The listing builds one solid part. Answer for the finished solid, in the listing's coordinates (mm). A direction names the side the tool comes from. Coordinates: 2 decimals unless noted, no trailing zeros. Write each loop counter-clockwise with the first axis right and the second up, starting at its lowest first coordinate (ties: lowest second). Pieces come first, ordered by that corner, then holes.
(1) Given P1, Ø2, axis at x = -7, y = 7.5, coming from the -Z side; P2, Ø1, axis at x = -7, z = 24, coming from the +Y side; P3, Ø1.3, axis at y = -4, z = 24, coming from the +X side; P4, Ø7, axis at x = -25, z = -3, coming from the -Y side, each flat-ended and moving along its own axis, determine where each tip first touches the part or whether it passes through.
(2) Which of the six approach directions +Z, -Z, +X, -X, +Y, -Y give full straight-line access (tool end or side, diameter ignored) to faces 1 (the flat face through (25, 0, 0)), 2 (the flat face through (0, 10.16, -19)), 3 (the cylindrical face through (0.827, 1.216, -24.148)), 4 (the flat face through (-7, 2.54, 24)), 5 (the flat face through (0, 10.16, 19))?
(3) Straight lines are drawn through the part: line 1 (Y direction, x = 0, z = 23.9); line 2 (X direction, y = 6.25, z = -5) (3 decimals); line 3 (Z direction, x = 6.5, y = -2). For each, find the intervals that lie inside material, in ascending order.
(4) The part is cut by section A-A on y = 5.5. Determine the outline of the cut face in (x, z) (3 decimals).
(5) For a pull along X with two mould halves and no side action, classify faces 6 (the flat face through (6.35, 6, 0)), 7 (the flat face through (-28, 2.54, 0)), 8 (the flat face through (-27.305, 8, 0)) as +X half, -X half, draft (parallel to the pull), parting line (faces both ways), or undercut.
(6) The part is cut by section C-C on z = 11.5. Determine the outline of the cut face in (x, y) (3 decimals).
(7) The part is cut by section D-D on y = -5.08. Determine the outline of the cut face in (x, z).
(8) The part is cut by section B-B on x = 0. Determine the outline of the cut face in (y, z), plus the area to 3 significant figures.
from build123d import *

# Parameters (mm, degrees)
SKETCH1_W           = 57.15
SKETCH1_H           = 25.4
BOSS_EXTRUDE1_DEPTH = 15.24
SKETCH2_W           = 44.45
SKETCH2_H           = 25.4
CUT_EXTRUDE1_DEPTH  = 10.16
SKETCH3_W           = 1.27
SKETCH3_H           = 10.16
CUT_EXTRUDE2_DEPTH  = 42.157602275
BOSS_EXTRUDE2_START = -10.16
SKETCH4_W           = 12.7
SKETCH4_H           = 50.8
BOSS_EXTRUDE2_DEPTH = 7.62
SKETCH6_W           = 15.24
SKETCH6_H           = 15.24
SKETCH6_R           = 6.35
BOSS_EXTRUDE3_DEPTH = 2.54


with BuildPart() as part:
    # Sketch1 → Boss-Extrude1 (new body)
    with BuildSketch(Plane(origin=(0, 0, 0), x_dir=(1, 0, 0), z_dir=(0, 1, 0))):
        Rectangle(SKETCH1_W, SKETCH1_H)
    extrude(amount=BOSS_EXTRUDE1_DEPTH)

    # Sketch2 → Cut-Extrude1 (cut)
    with BuildSketch(Plane.XZ):
        Rectangle(SKETCH2_W, SKETCH2_H)
    extrude(amount=-CUT_EXTRUDE1_DEPTH, mode=Mode.SUBTRACT)

    # Sketch3 → Cut-Extrude2 (cut, through all)
    with BuildSketch(Plane.XY.offset(12.7)):
        with Locations((-27.94, 7.62)):
            Rectangle(SKETCH3_W, SKETCH3_H)
        with Locations((27.94, 7.62)):
            Rectangle(SKETCH3_W, SKETCH3_H)
    extrude(amount=-CUT_EXTRUDE2_DEPTH, mode=Mode.SUBTRACT)

    # Sketch4 → Boss-Extrude2 (add)
    with BuildSketch(Plane.XZ.offset(BOSS_EXTRUDE2_START)):
        Rectangle(SKETCH4_W, SKETCH4_H)
    extrude(amount=BOSS_EXTRUDE2_DEPTH)

    # Sketch6 → Boss-Extrude3 (add)
    with BuildSketch(Plane(origin=(0, 0, -25.4), x_dir=(-1, 0, 0), z_dir=(0, 0, -1))):
        with Locations((0, -5.08)):
            Rectangle(SKETCH6_W, SKETCH6_H)
        with Locations((0, -5.08)):
            Circle(SKETCH6_R, mode=Mode.SUBTRACT)
    boss_extrude3 = extrude(amount=-BOSS_EXTRUDE3_DEPTH)

    # Mirror1: Boss-Extrude3 across plane
    add(boss_extrude3.mirror(Plane.XY))


solid = part.part
Model answer:
1. P1: stops at z = -25.4
1. P2: stops at y = 2.54
1. P3: stops at x = 7.62
1. P4: stops at y = 0
2. face 1: +Z, -Z, +X, -X, -Y
2. face 2: -Z, +X, -X, +Y
2. face 3: +Z, -Z
2. face 4: +Z, -Z, -X, +Y
2. face 5: +Z, +X, -X, +Y
3. line 1: y = -12.7 to -11.43, 1.27 to 10.16
3. line 2: x = -27.305 to -22.225, -6.35 to 6.35, 22.225 to 27.305
3. line 3: z = -25.4 to -22.86, 22.86 to 25.4
4. outline: (-27.305, -12.7) - (-22.225, -12.7) - (-22.225, 12.7) - (-27.305, 12.7) - close; (-6.35, -25.4) - (6.35, -25.4) - (6.35, 25.4) - (-6.35, 25.4) - close; (22.225, -12.7) - (27.305, -12.7) - (27.305, 12.7) - (22.225, 12.7) - close
5. face 6: undercut
5. face 7: draft
5. face 8: -X half
6. outline: (-28.575, 0) - (-22.225, 0) - (-22.225, 10.16) - (-6.35, 10.16) - (-6.35, 2.54) - (6.35, 2.54) - (6.35, 10.16) - (22.225, 10.16) - (22.225, 0) - (28.575, 0) - (28.575, 2.54) - (27.305, 2.54) - (27.305, 12.7) - (28.575, 12.7) - (28.575, 15.24) - (-28.575, 15.24) - (-28.575, 12.7) - (-27.305, 12.7) - (-27.305, 2.54) - (-28.575, 2.54) - close
7. outline: (-7.62, -25.4) - (-6.35, -25.4) - (-6.35, -22.86) - (-7.62, -22.86) - close; (-7.62, 22.86) - (-6.35, 22.86) - (-6.35, 25.4) - (-7.62, 25.4) - close; (6.35, -25.4) - (7.62, -25.4) - (7.62, -22.86) - (6.35, -22.86) - close; (6.35, 22.86) - (7.62, 22.86) - (7.62, 25.4) - (6.35, 25.4) - close
8. outline: (-12.7, -25.4) - (-11.43, -25.4) - (-11.43, -22.86) - (-12.7, -22.86) - close; (-12.7, 22.86) - (-11.43, 22.86) - (-11.43, 25.4) - (-12.7, 25.4) - close; (1.27, -25.4) - (10.16, -25.4) - (10.16, -12.7) - (15.24, -12.7) - (15.24, 12.7) - (10.16, 12.7) - (10.16, 25.4) - (1.27, 25.4) - (1.27, 22.86) - (2.54, 22.86) - (2.54, -22.86) - (1.27, -22.86) - close
8. area: 529 mm2
